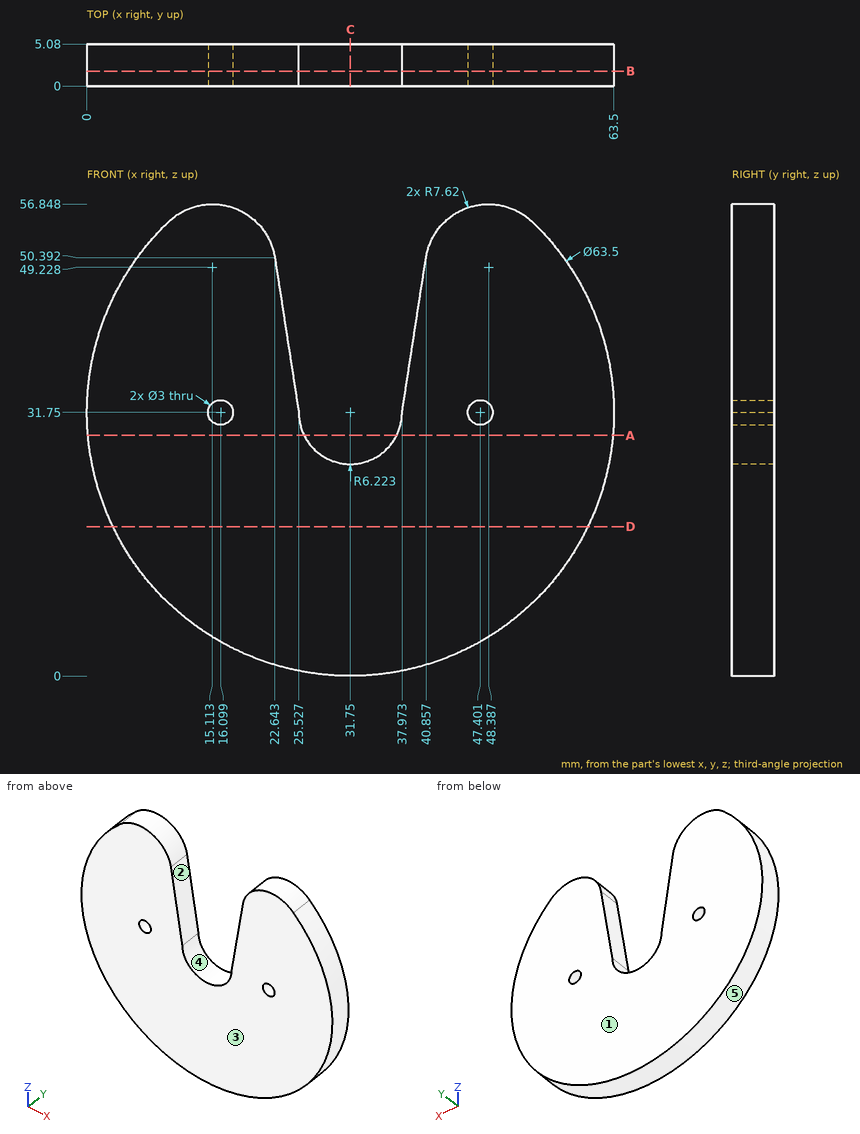
Verification items for this drawing (mm, ordinates from the low corner). A direction names the side the tool comes from. Give positions to 0.01 mm unless a question says otherwise; leave off trailing zeros. Loops run counter-clockwise (first coordinate to the right, second up) from the corner with the lowest first, then second, coordinate; pieces in that order, holes last.
1. Cross-section at A-A on z = 29. Record the cut outline in (x, y), and give its area (3 significant figures).
Derived:
outline: (0.12, 0) - (26.17, 0) - (26.17, 5.08) - (0.12, 5.08) - close; (37.33, 0) - (63.38, 0) - (63.38, 5.08) - (37.33, 5.08) - close
area: 265 mm2
2. Cross-section at C-C on x = 31.75. Record the cut outline in (y, z), and give its area (3 significant figures).
Derived:
outline: (0, 0) - (5.08, 0) - (5.08, 25.53) - (0, 25.53) - close
area: 130 mm2
3. Release check for a two-part mould opening along X. For the marked faces 3, 4 and 5 record: +X half, -X half, draft (parallel to the pull), parting line (faces both ways), or undercut.
Derived:
face 3: draft
face 4: undercut
face 5: parting line
4. Cross-section at D-D on z = 18. Record the cut outline in (x, y).
Derived:
outline: (3.13, 0) - (60.37, 0) - (60.37, 5.08) - (3.13, 5.08) - close
5. Cross-section at B-B on y = 1.8. Record the cut outline in (x, z), and give its area (3 significant figures).
Derived:
outline: (9.86, 54.75) arc R31.75 ccw (long way) to (53.64, 54.75) arc R7.62 ccw to (40.86, 50.39) - (37.97, 31.75) arc R6.22 cw to (25.53, 31.75) - (22.64, 50.39) arc R7.62 ccw to start; hole circle Ø3 at (16.1, 31.75); hole circle Ø3 at (47.4, 31.75)
area: 2,490 mm2
6. Go/stop test with flat-tipped pins: P1, Ø3, axis at x = 25, y = 3, coming from the -Z side; P2, Ø2, axis at y = 3.5, z = 28.5, coming from the -X side. Record where each tip stops, or that it passes through.
Derived:
P1: stops at z = 0.44
P2: stops at x = 0.08
7. Tool access check on the marked faces 1 and 2. Record the directions out of +Z, -Z, +X, -X, +Y, -Y that give a thin tool (end or side, any length) a straight path to the whole face; none if there is none.
Derived:
face 1: +Z, -Z, +X, -X, +Y
face 2: +Z, +Y, -Y
8. Material ranges on probe 1 along Z at (x, y) = (16.5, 0.95) (1 decimal); probe 2 along X at (y, z) = (1.6, 30.5) (1 decimal); probe 3 along X at (y, z) = (1.7, 51) (1 decimal), recorded low to high.
Derived:
probe 1: z = 3.9 to 30.3, 33.2 to 56.7
probe 2: x = 0 to 15.3, 16.9 to 25.7, 37.8 to 46.6, 48.2 to 63.5
probe 3: x = 6.5 to 22.5, 41 to 57
